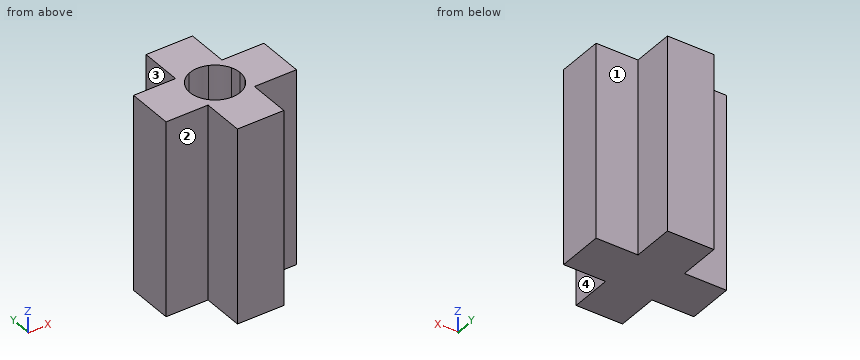
from build123d import *

# Parameters (mm, degrees)
F1_DEPTH = 7.7724
F2_DEPTH = 2.54


with BuildPart() as f1:
    # F0 (on Top) → F1 (new body)
    with BuildSketch(Plane.XY):
        with BuildLine():
            Line((29.3928639389, -5.0019352848), (29.3928639389, -6.6783352848))
            Line((29.3928639389, -6.6783352848), (29.9364323496, -6.6783352848))
            ThreePointArc((29.9364323496, -6.6783352848), (30.3199639389, -6.6021352848), (30.7034955282, -6.6783352848))
            Line((30.7034955282, -6.6783352848), (31.2470639389, -6.6783352848))
            Line((31.2470639389, -6.6783352848), (31.2470639389, -5.0019352848))
            Line((31.2470639389, -5.0019352848), (29.3928639389, -5.0019352848))
        make_face()
        with BuildLine():
            Line((29.9364323496, -6.6783352848), (29.3928639389, -6.6783352848))
            Line((29.3928639389, -6.6783352848), (29.3928639389, -7.2219036954))
            ThreePointArc((29.3928639389, -7.2219036954), (29.6105237053, -6.8959950512), (29.9364323496, -6.6783352848))
        make_face()
        with BuildLine():
            Line((29.3928639389, -6.6783352848), (27.7164639389, -6.6783352848))
            Line((27.7164639389, -6.6783352848), (27.7164639389, -8.5325352848))
            Line((27.7164639389, -8.5325352848), (29.3928639389, -8.5325352848))
            Line((29.3928639389, -8.5325352848), (29.3928639389, -7.9889668741))
            ThreePointArc((29.3928639389, -7.9889668741), (29.3166639389, -7.6054352848), (29.3928639389, -7.2219036954))
            Line((29.3928639389, -7.2219036954), (29.3928639389, -6.6783352848))
        make_face()
        with BuildLine():
            Line((29.9364323496, -8.5325352848), (29.3928639389, -8.5325352848))
            Line((29.3928639389, -8.5325352848), (29.3928639389, -10.2089352848))
            Line((29.3928639389, -10.2089352848), (31.2470639389, -10.2089352848))
            Line((31.2470639389, -10.2089352848), (31.2470639389, -8.5325352848))
            Line((31.2470639389, -8.5325352848), (30.7034955282, -8.5325352848))
            ThreePointArc((30.7034955282, -8.5325352848), (30.3199639389, -8.6087352848), (29.9364323496, -8.5325352848))
        make_face()
        with BuildLine():
            Line((32.9234639389, -6.6783352848), (31.2470639389, -6.6783352848))
            Line((31.2470639389, -6.6783352848), (31.2470639389, -7.2219036954))
            ThreePointArc((31.2470639389, -7.2219036954), (31.3040295668, -7.4099212699), (31.3232639389, -7.6054352848))
            ThreePointArc((31.3232639389, -7.6054352848), (31.3040295668, -7.8009492996), (31.2470639389, -7.9889668741))
            Line((31.2470639389, -7.9889668741), (31.2470639389, -8.5325352848))
            Line((31.2470639389, -8.5325352848), (32.9234639389, -8.5325352848))
            Line((32.9234639389, -8.5325352848), (32.9234639389, -6.6783352848))
        make_face()
        with BuildLine():
            Line((31.2470639389, -6.6783352848), (30.7034955282, -6.6783352848))
            ThreePointArc((30.7034955282, -6.6783352848), (31.0294041725, -6.8959950512), (31.2470639389, -7.2219036954))
            Line((31.2470639389, -7.2219036954), (31.2470639389, -6.6783352848))
        make_face()
        with BuildLine():
            ThreePointArc((31.2470639389, -7.9889668741), (31.0294041725, -8.3148755183), (30.7034955282, -8.5325352848))
            Line((30.7034955282, -8.5325352848), (31.2470639389, -8.5325352848))
            Line((31.2470639389, -8.5325352848), (31.2470639389, -7.9889668741))
        make_face()
        with BuildLine():
            Line((29.3928639389, -7.9889668741), (29.3928639389, -8.5325352848))
            Line((29.3928639389, -8.5325352848), (29.9364323496, -8.5325352848))
            ThreePointArc((29.9364323496, -8.5325352848), (29.6105237053, -8.3148755183), (29.3928639389, -7.9889668741))
        make_face()
    extrude(amount=F1_DEPTH)

    # F0 (on Top) → F2 (join)
    with BuildSketch(Plane.XY):
        with BuildLine():
            Line((30.7034955282, -6.6783352848), (29.9364323496, -6.6783352848))
            ThreePointArc((29.9364323496, -6.6783352848), (29.6105237053, -6.8959950512), (29.3928639389, -7.2219036954))
            Line((29.3928639389, -7.2219036954), (29.3928639389, -7.9889668741))
            ThreePointArc((29.3928639389, -7.9889668741), (29.6105237053, -8.3148755183), (29.9364323496, -8.5325352848))
            Line((29.9364323496, -8.5325352848), (30.7034955282, -8.5325352848))
            ThreePointArc((30.7034955282, -8.5325352848), (31.0294041725, -8.3148755183), (31.2470639389, -7.9889668741))
            Line((31.2470639389, -7.9889668741), (31.2470639389, -7.2219036954))
            ThreePointArc((31.2470639389, -7.2219036954), (31.0294041725, -6.8959950512), (30.7034955282, -6.6783352848))
        make_face()
        with BuildLine():
            Line((29.3928639389, -7.9889668741), (29.3928639389, -7.2219036954))
            ThreePointArc((29.3928639389, -7.2219036954), (29.3166639389, -7.6054352848), (29.3928639389, -7.9889668741))
        make_face()
        with BuildLine():
            Line((30.7034955282, -8.5325352848), (29.9364323496, -8.5325352848))
            ThreePointArc((29.9364323496, -8.5325352848), (30.3199639389, -8.6087352848), (30.7034955282, -8.5325352848))
        make_face()
        with BuildLine():
            ThreePointArc((31.3232639389, -7.6054352848), (31.3040295668, -7.4099212699), (31.2470639389, -7.2219036954))
            Line((31.2470639389, -7.2219036954), (31.2470639389, -7.9889668741))
            ThreePointArc((31.2470639389, -7.9889668741), (31.3040295668, -7.8009492996), (31.3232639389, -7.6054352848))
        make_face()
        with BuildLine():
            ThreePointArc((30.7034955282, -6.6783352848), (30.3199639389, -6.6021352848), (29.9364323496, -6.6783352848))
            Line((29.9364323496, -6.6783352848), (30.7034955282, -6.6783352848))
        make_face()
    extrude(amount=F2_DEPTH)


solid = f1.part
Work out the finished part from the listing and answer in its coordinate system (mm). Face numbers are marked on the shaded views. A direction names the side the tool comes from. Give positions to 0.01 mm unless a question says otherwise; leave off trailing zeros. Loops run counter-clockwise (first coordinate to the right, second up) from the corner with the lowest first, then second, coordinate; pieces in that order, holes last. Notation, with made-up numbers: M 71.5,18.5 L 78.5,18.5 A16 cw 78.5,45.5 Z; hole C 44,58.25 d11. An arc over 180 degrees is marked long. Use CSV: the item, a comma, the result in double quotes.
1) Which of the six approach directions +Z, -Z, +X, -X, +Y, -Y give full straight-line access (tool end or side, diameter ignored) to the marked faces 1, 2, 3 and 4?
Answer:
face 1,"+Z, -Z, +X, +Y"
face 2,"+Z, -Z, -X, -Y"
face 3,"+Z, -Z, -X, +Y"
face 4,"+Z, -Z, +X, -Y"
2) Consider L1, parallel to Y at x = 31.4, z = 3.5; L2, parallel to X at y = -5.85, z = 5; L3, parallel to Z at x = 31.1, y = -7.1. Determine where each line is inside the solid, lowest interval first.
Answer:
L1,"-8.53 to -6.68"
L2,"29.39 to 31.25"
L3,"0 to 2.54"
3) Given P1, Ø1.8, axis at y = -6, z = 5.5, coming from the +X side; P2, Ø1.5, axis at y = -5.5, z = 3.5, coming from the -X side; P3, Ø0.5, axis at x = 32, z = 5.5, coming from the +Y side; P4, Ø1.8, axis at y = -9.5, z = 5, coming from the +X side, each flat-ended and moving along its own axis, determine where each tip first touches the part or whether it passes through.
Answer:
P1,"x = 32.92"
P2,"x = 29.39"
P3,"y = -6.68"
P4,"x = 31.25"
4) Find section C-C on x = 30.5. Write down the section's boundary in (y, z).
Answer:
outline,"M -10.21,0 L -5,0 L -5,7.77 L -6.62,7.77 L -6.62,2.54 L -8.59,2.54 L -8.59,7.77 L -10.21,7.77 Z"
5) Find section A-A on z = 3. Write down the section's boundary in (x, y).
Answer:
outline,"M 27.72,-8.53 L 29.39,-8.53 L 29.39,-10.21 L 31.25,-10.21 L 31.25,-8.53 L 32.92,-8.53 L 32.92,-6.68 L 31.25,-6.68 L 31.25,-5 L 29.39,-5 L 29.39,-6.68 L 27.72,-6.68 Z; hole C 30.32,-7.61 d2.01"
6) Find section B-B on z = 0.5. Write down the section's boundary in (x, y).
Answer:
outline,"M 27.72,-8.53 L 29.39,-8.53 L 29.39,-10.21 L 31.25,-10.21 L 31.25,-8.53 L 32.92,-8.53 L 32.92,-6.68 L 31.25,-6.68 L 31.25,-5 L 29.39,-5 L 29.39,-6.68 L 27.72,-6.68 Z"
7) Find section D-D on y = -6. Write down the section's boundary in (x, z).
Answer:
outline,"M 29.39,0 L 31.25,0 L 31.25,7.77 L 29.39,7.77 Z"
